For this review, take the finished solid that the model builds, in its own axes (mm). A direction names the side the tool comes from. Give positions to 0.01 mm unless a question says otherwise; leave off trailing zeros. Loops run counter-clockwise (first coordinate to the right, second up) from the corner with the lowest first, then second, coordinate; pieces in that order, holes last. Notation, with made-up numbers: (-37.5, -8) - (-12.5, -8) arc R29 cw to (-12.5, 18) - close; hole circle Ø3 at (40.5, 43.25). An arc over 180 degrees is marked (long way). Answer in a Markdown table with one row per item.
```python
from build123d import *

# Parameters (mm, degrees)
BOSS_EXTRUDE1_DEPTH     = 7.5
CUT_EXTRUDE1_DEPTH      = 41.233692349
CUT_EXTRUDE1_DEPTH_BACK = 41.233692349
SKETCH3_R               = 4.7625
FILLET1_R               = 7.5
F_8_32_TAPPED_HOLE1_D   = 3.4544


with BuildPart() as part:
    # Sketch1 → Boss-Extrude1 (new, symmetric)
    with BuildSketch(Plane(origin=(0, 0, 0), x_dir=(1, 0, 0), z_dir=(0, 1, 0))):
        Polygon((-17.5, -7.5), (-22.5, -7.5), (-22.5, 32.5), (22.5, 32.5), (22.5, -7.5), (17.5, -7.5), (17.5, 27.5), (-17.5, 27.5), align=None)
    extrude(amount=BOSS_EXTRUDE1_DEPTH, both=True)

    # Sketch3 → Cut-Extrude1 (cut, two sides: drawn at the far end of the back side and taken through both)
    with BuildSketch(Plane(origin=(0, 0, 0), x_dir=(0, 0, -1), z_dir=(1, 0, 0)).offset(-CUT_EXTRUDE1_DEPTH_BACK)):
        Circle(SKETCH3_R)
    extrude(amount=CUT_EXTRUDE1_DEPTH + CUT_EXTRUDE1_DEPTH_BACK, mode=Mode.SUBTRACT)

    # Fillet1
    fillet1_edges = [part.edges().sort_by_distance(p)[0] for p in [
        (20, 7.5, 7.5),
        (20, -7.5, 7.5),
        (-20, -7.5, 7.5),
        (-20, 7.5, 7.5),
    ]]
    fillet(fillet1_edges, radius=FILLET1_R - 0.0001)  # a hair under: the kernel refuses the full size

    # #8-32 Tapped Hole1 (through all)
    with Locations(Plane.XY.offset(-27.5)):
        with Locations((-13.47, 0)):
            Hole(F_8_32_TAPPED_HOLE1_D / 2)


solid = part.part
```
1. We need section B-B, the plane z = -10. Give the boundary of the cut face in (x, y).
Values:
| item | result |
|---|---|
| outline | (-22.5, -7.5) - (-17.5, -7.5) - (-17.5, 7.5) - (-22.5, 7.5) - close; (17.5, -7.5) - (22.5, -7.5) - (22.5, 7.5) - (17.5, 7.5) - close |
2. Clearance check with flat-ended pins moving along their axes: pin 1 (6 mm diameter, centred on y = 3.5, z = 0.5, fed in from +X); pin 2 (5 mm diameter, centred on x = -7, y = -2.5, fed in from +Z); pin 3 (7.5 mm diameter, centred on y = 0, z = 0, fed in from +X). State where each tip first meets the part, or that it passes through.
Values:
| item | result |
|---|---|
| pin 1 | stops at x = 22.5 |
| pin 2 | stops at z = -27.5 |
| pin 3 | passes through |
3. Mouldability with a two-part tool opening along X and no side actions: class faces 3 (the face through (19.965, -5.361, 5.245)), 4 (the face through (0, 0, -27.5)), 5 (the face through (22.5, 0, -13)), 6 (the face through (-22.5, 0, -17)) as released by +X, released by -X, zero draft, split by the parting line, or undercut.
Values:
| item | result |
|---|---|
| face 3 | zero draft |
| face 4 | undercut |
| face 5 | released by +X |
| face 6 | released by -X |
4. We need section C-C, the plane y = -6.5. Give the boundary of the cut face in (x, z).
Values:
| item | result |
|---|---|
| outline | (-22.5, -32.5) - (22.5, -32.5) - (22.5, 3.74) - (17.5, 3.74) - (17.5, -27.5) - (-17.5, -27.5) - (-17.5, 3.74) - (-22.5, 3.74) - close |
5. For faces 1 (the face through (19.96, -2.9, 3.78)), 2 (the face through (17.5, 0, -14)), list the 3-axis set-ups (+Z, -Z, +X, -X, +Y, -Y) from which the entire face can be reached by the end or side of a thin tool; tool diameter is ignored.
Values:
| item | result |
|---|---|
| face 1 | +X, -X |
| face 2 | +Z, +Y, -Y |
6. We need section A-A, the plane x = -13.47. Give the boundary of the cut face in (y, z).
Values:
| item | result |
|---|---|
| outline | (-7.5, -32.5) - (-1.73, -32.5) - (-1.73, -27.5) - (-7.5, -27.5) - close; (1.73, -32.5) - (7.5, -32.5) - (7.5, -27.5) - (1.73, -27.5) - close |
7. We need section D-D, the plane y = 5.5. Give the boundary of the cut face in (x, z), and give its area (3 significant figures).
Values:
| item | result |
|---|---|
| outline | (-22.5, -32.5) - (22.5, -32.5) - (22.5, 5.1) - (17.5, 5.1) - (17.5, -27.5) - (-17.5, -27.5) - (-17.5, 5.1) - (-22.5, 5.1) - close |
| area | 551 mm^2 |
8. Wall thickness on line 1 (X direction, y = 1, z = -24); line 2 (Z direction, x = 20.55, y = 0); line 3 (Z direction, x = 14.5, y = -5): over which ranges is each line inside the solid? List them lowest first. Write a range as [from, to].
Values:
| item | result |
|---|---|
| line 1 | x = [-22.5, -17.5], [17.5, 22.5] |
| line 2 | z = [-32.5, -4.76], [4.76, 7.5] |
| line 3 | z = [-32.5, -27.5] |
